Job drawing, mm, ordinate dimensions from the low corner. One solid piece. A direction names the side the tool comes from. Round coordinates to 2 decimals unless told otherwise and drop trailing zeros. Loops run counter-clockwise (first coordinate to the right, second up) from the corner with the lowest first, then second, coordinate; pieces in that order, holes last. Notation, with made-up numbers: (61, -4) - (79, -4) arc R22 ccw to (79, 29) - close; hole circle Ø7 at (59.25, 58.5). An arc over 180 degrees is marked (long way). One line per question, with ' | ' between items. Start each with the question number.
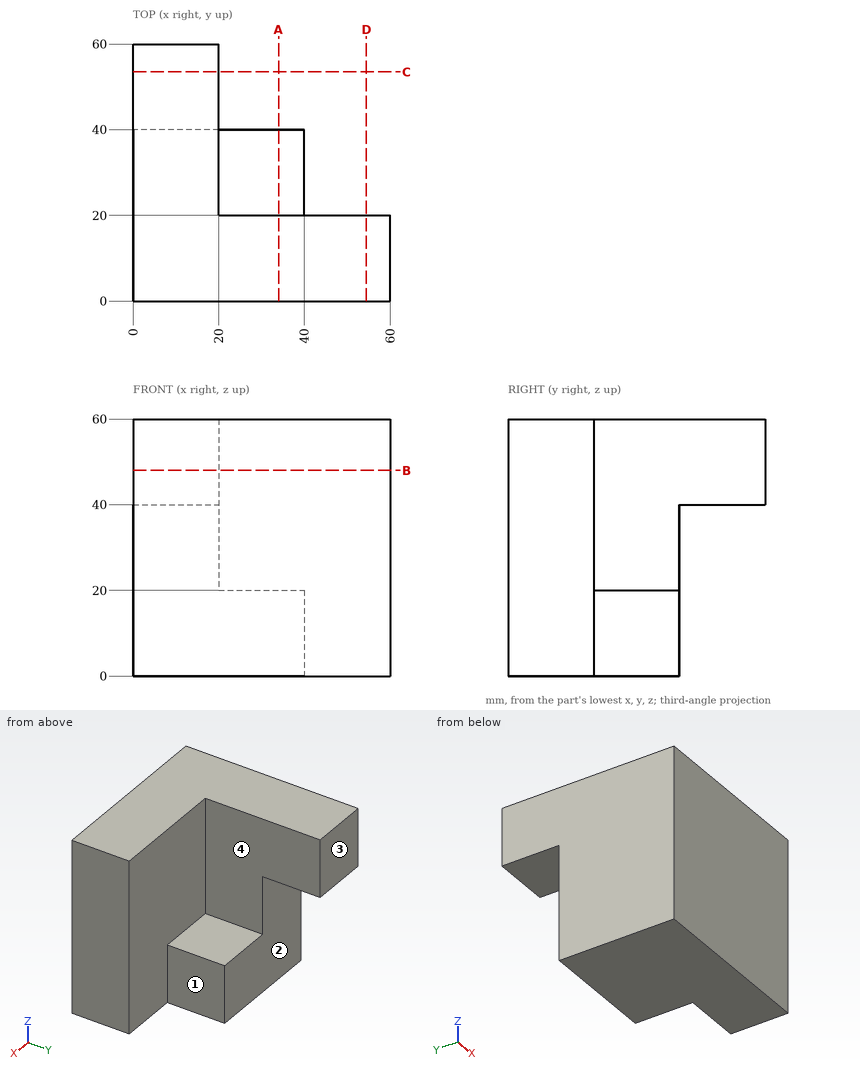
1) Saw through at C-C on y = 53.5. Write the cut outline in (x, z), and give its area (3 significant figures).
2) Wall check: line 1 (Z direction, x = 35, y = 20.5); line 2 (Y direction, x = 15.5, z = 29). Give the ranges that are in metal, low to high. Write a range as [from, to].
3) Saw through at D-D on x = 54.5. Write the cut outline in (y, z).
4) Saw through at A-A on x = 34. Write the cut outline in (y, z), and give its area (3 significant figures).
5) Drop flat-ended pins along their axis: pin 1 (12 mm diameter, centred on y = 32, z = 31, fed in from +X); pin 2 (6 mm diameter, centred on x = 40.5, y = 44.5, fed in from -Z); pin 3 (16 mm diameter, centred on y = 33, z = 14.5, fed in from +X); pin 4 (10 mm diameter, centred on x = 10, y = 50, fed in from -Z). Give the stop position or say it passes through.
6) Tool access for the marked faces 1, 2, 3 and 4: list every direction of +Z, -Z, +X, -X, +Y, -Y with a clear straight run to the whole face (end or side of a thin tool).
7) Saw through at B-B on z = 48. Write the cut outline in (x, y).
Answer key:
1) outline: (0, 40) - (20, 40) - (20, 60) - (0, 60) - close | area: 400 mm²
2) line 1: [0, 20] | line 2: [0, 40]
3) outline: (0, 0) - (20, 0) - (20, 60) - (0, 60) - close
4) outline: (0, 0) - (40, 0) - (40, 20) - (20, 20) - (20, 60) - (0, 60) - close | area: 1,600 mm²
5) pin 1: x = 20 | pin 2: through | pin 3: x = 40 | pin 4: z = 40
6) face 1: +Z, -Z, +X, +Y | face 2: -Z, +X, -X, +Y | face 3: +Z, -Z, +X, -X, +Y | face 4: +Z, +X, +Y
7) outline: (0, 0) - (60, 0) - (60, 20) - (20, 20) - (20, 60) - (0, 60) - close
